The model under review builds one solid part; all positions refer to its coordinate system, in mm. A direction names the side the tool comes from. Give positions to 0.01 mm unless a question says otherwise; leave off trailing zeros. Order: outer loops, then holes, each group sorted by start corner. A loop starts at its lowest first (then second) coordinate and runs counter-clockwise, first axis right, second up. Notation, with made-up numbers: (83.25, 0) - (99.25, 0) arc R28 ccw to (99.25, 20) - close; hole circle Ø6 at (74.5, -18.75). An arc over 180 degrees is marked (long way). Write item = value, one per line. Start each with the question number.
1. We need section D-D, the plane z = 8. Give the boundary of the cut face in (x, y), and give its area (3 significant figures).
2. We need section C-C, the plane z = 10.75. Give the boundary of the cut face in (x, y), and give its area (3 significant figures).
3. Machinability: for faces 1 (the flat face through (-1, 7, 25.146)), 2 (the cylindrical face through (-0.77, 17.27, 12.52)), 3 (the flat face through (-1.524, 11.3, 9.6)), which of the approach directions +Z, -Z, +X, -X, +Y, -Y give a long, thin tool a straight path to every point of the face, cutting with its end or side? Answer none if there is none.
4. We need section B-B, the plane x = -7. Give the boundary of the cut face in (y, z), and give its area (3 significant figures).
5. Mouldability with a two-part tool opening along X and no side actions: class faces 4 (the cylindrical face through (-0.773, 4.573, 12.629)), 5 (the flat face through (0, 10.3, 9.6)), 6 (the cylindrical face through (-7.9, 0.77, 10.32)) as pulls with the +X half, pulls with the -X half, needs draft (parallel to the pull), parting line crosses it, or undercut.
6. For P1, Ø9.5, axis at y = 7.5, z = 16.5, coming from the -X side; P2, Ø8, axis at x = -7.5, z = 7.5, coming from the -Y side, all flat-tipped, find the tip position at first contact; note any pin that passes through.
7. Wall thickness on probe 1 along X at (y, z) = (9.75, 22); probe 2 along Y at (x, z) = (-3.5, 21.75); probe 3 along Y at (x, z) = (-1, 11): over which ranges is each line inside the solid? List them lowest first.
8. We need section A-A, the plane y = 8.5. Give the boundary of the cut face in (x, z), and give its area (3 significant figures).
from build123d import *

# Parameters (mm, degrees)
BOSS_EXTRUDE2_DEPTH = 25.146
CUT_EXTRUDE1_REACH  = 37.415
CUT_EXTRUDE2_REACH  = 37.174
SKETCH4_R           = 2.54


with BuildPart() as part:
    # Sketch1 → Boss-Extrude2 (new body)
    with BuildSketch(Plane.XY):
        Polygon((-15.24, 0), (0, 0), (0, 20.828), (-1.524, 20.828), (-1.524, 1.524), (-15.24, 1.524), align=None)
    extrude(amount=BOSS_EXTRUDE2_DEPTH)

    # Sketch3 → Cut-Extrude1 (cut, up to next)
    with BuildSketch(Plane.ZY.offset(1.524), mode=Mode.PRIVATE) as cut_extrude1_sk1:
        with BuildLine():
            Line((15.113, 14.732), (15.113, 7.112))
            ThreePointArc((15.113, 7.112), (12.573, 4.572), (10.033, 7.112))
            Line((10.033, 7.112), (10.033, 14.732))
            ThreePointArc((10.033, 14.732), (12.573, 17.272), (15.113, 14.732))
        make_face()
    cut_extrude1_tool1 = extrude(cut_extrude1_sk1.sketch, amount=-CUT_EXTRUDE1_REACH, mode=Mode.PRIVATE) & part.part
    add(cut_extrude1_tool1.solids().sort_by_distance((-1.524, 10.922, 12.573))[0], mode=Mode.SUBTRACT)

    # Sketch4 → Cut-Extrude2 (cut, up to next)
    with BuildSketch(Plane(origin=(0, 1.524, 0), x_dir=(1, 0, 0), z_dir=(0, 1, 0)), mode=Mode.PRIVATE) as cut_extrude2_sk1:
        with Locations(Location((-6.731, -12.573, 0), (0, 0, 180))):
            Circle(SKETCH4_R)
    cut_extrude2_tool1 = extrude(cut_extrude2_sk1.sketch, amount=-CUT_EXTRUDE2_REACH, mode=Mode.PRIVATE) & part.part
    add(cut_extrude2_tool1.solids().sort_by_distance((-6.731, 1.524, 12.573))[0], mode=Mode.SUBTRACT)


solid = part.part
Model answer:
q1.outline = (-15.24, 0) - (0, 0) - (0, 20.83) - (-1.52, 20.83) - (-1.52, 1.52) - (-15.24, 1.52) - close
q1.area = 52.6 mm2
q2.outline = (-15.24, 0) - (-8.5, 0) - (-8.5, 1.52) - (-15.24, 1.52) - close; (-4.96, 0) - (0, 0) - (0, 5.34) - (-1.52, 5.34) - (-1.52, 1.52) - (-4.96, 1.52) - close; (-1.52, 16.5) - (0, 16.5) - (0, 20.83) - (-1.52, 20.83) - close
q2.area = 30.3 mm2
q3.face_1 = +Z, +X, -X, +Y, -Y
q3.face_2 = +X, -X
q3.face_3 = +Z, -Z, -X, +Y
q4.outline = (0, 0) - (1.52, 0) - (1.52, 10.05) - (0, 10.05) - close; (0, 15.1) - (1.52, 15.1) - (1.52, 25.15) - (0, 25.15) - close
q4.area = 30.6 mm2
q5.face_4 = needs draft
q5.face_5 = pulls with the +X half
q5.face_6 = undercut
q6.P1 = -1.52
q6.P2 = 0
q7.probe_1 = -1.52 to 0
q7.probe_2 = 0 to 1.52
q7.probe_3 = 0 to 5.12, 16.73 to 20.83
q8.outline = (-1.52, 0) - (0, 0) - (0, 10.03) - (-1.52, 10.03) - close; (-1.52, 15.11) - (0, 15.11) - (0, 25.15) - (-1.52, 25.15) - close
q8.area = 30.6 mm2
